Study the drawing (mm; zero at the part's minimum x, y, z) and answer. A direction names the side the tool comes from. Give positions to 0.01 mm unless a question says otherwise; leave off trailing zeros. Loops run counter-clockwise (first coordinate to the right, second up) from the corner with the lowest first, then second, coordinate; pieces in that order, holes last. Notation, with made-up numbers: (15, -12.5) - (44, -12.5) arc R17 cw to (44, 6.5) - close; hole circle Ø4 at (39, 61.5). An arc over 180 degrees is marked (long way). Write item = value, one per line. Start each with the question number.
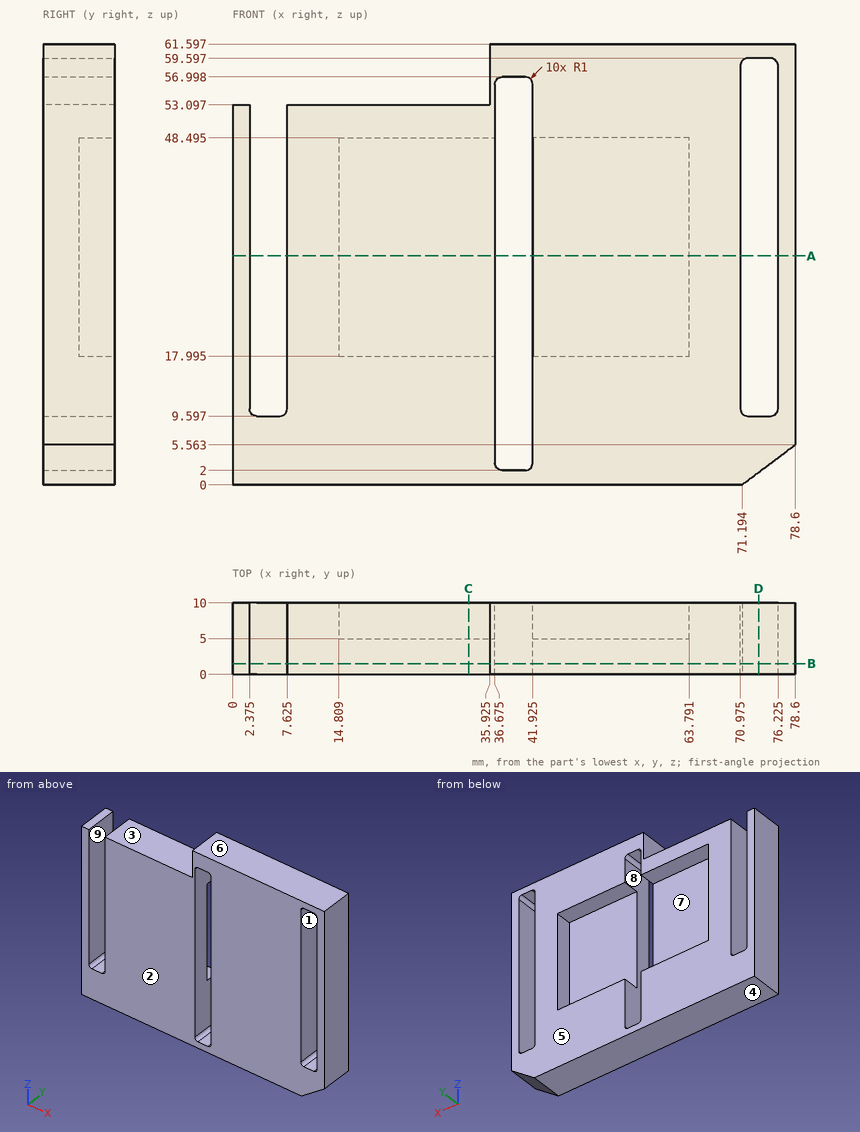
1. Consider line 1 along X through (y, z) = (8.75, 26) (1 decimal); line 2 along X through (y, z) = (2.75, 30.5) (1 decimal); line 3 along Z through (x, y) = (40.5, 7). Determine where each line is inside the solid, lowest interval first. Write a range as [from, to].
2. A cutting plane is placed at A-A on z = 32. Give the vertices of the cut face in (x, y) (1 decimal), and give its area (3 significant figures).
3. For a pull along Z with two mould halves and no side action, classify the marked faces 1, 2, 3 and 4 as released by +Z, released by -Z, zero draft, split by the parting line, or undercut.
4. A cutting plane is placed at D-D on x = 73.5. Give the vertices of the cut face in (y, z).
5. A cutting plane is placed at B-B on y = 1.5. Give the number of separate pieces and of enclosed holes in the cut face, and give its area (3 significant figures).
6. A cutting plane is placed at C-C on x = 33. Give the vertices of the cut face in (y, z) (1 decimal).
7. Given P1, Ø6.5, axis at x = 27.5, z = 40.5, coming from the +Y side; P2, Ø5.5, axis at x = 21.5, y = 6.5, coming from the +Z side; P3, Ø1.6, axis at x = 5.5, y = 6, coming from the +Z side; P4, Ø8, axis at x = 54.5, z = 55, coming from the -Y side, each flat-ended and moving along its own axis, determine where each tip first touches the part or whether it passes through.
8. A tool of negligible diameter and unlimited length cuts with its end or side. For the marked faces 5, 6, 7, 8 and 9, from which of +Z, -Z, +X, -X, +Y, -Y can it reach the whole face along a straight path? Write none if from no direction.
Reply:
q1.line_1 = [0, 2.4], [7.6, 14.8], [63.8, 71], [76.2, 78.6]
q1.line_2 = [0, 2.4], [7.6, 36.7], [41.9, 71], [76.2, 78.6]
q1.line_3 = [0, 2], [57, 61.6]
q2.outline = (0, 0) - (2.4, 0) - (2.4, 10) - (0, 10) - close; (7.6, 0) - (36.7, 0) - (36.7, 5) - (14.8, 5) - (14.8, 10) - (7.6, 10) - close; (41.9, 0) - (71, 0) - (71, 10) - (63.8, 10) - (63.8, 5) - (41.9, 5) - close; (76.2, 0) - (78.6, 0) - (78.6, 10) - (76.2, 10) - close
q2.area = 410 mm^2
q3.face_1 = undercut
q3.face_2 = zero draft
q3.face_3 = released by +Z
q3.face_4 = released by -Z
q4.outline = (0, 1.73) - (10, 1.73) - (10, 9.6) - (0, 9.6) - close; (0, 59.6) - (10, 59.6) - (10, 61.6) - (0, 61.6) - close
q5.separate_pieces = 1
q5.enclosed_holes = 2
q5.area = 3,740 mm^2
q6.outline = (0, 0) - (10, 0) - (10, 18) - (5, 18) - (5, 48.5) - (10, 48.5) - (10, 53.1) - (0, 53.1) - close
q7.P1 = 5
q7.P2 = 53.1
q7.P3 = 9.6
q7.P4 = 0
q8.face_5 = +Z, -Z, +X, -X, +Y
q8.face_6 = +Z, +X, -X, +Y, -Y
q8.face_7 = +Y
q8.face_8 = +Y, -Y
q8.face_9 = +Z, +Y, -Y
